Source: CAD feature listing. Evaluate the final solid. Frame: model axes, mm. A direction names the side the tool comes from. Give positions to 0.01 mm unless a question says otherwise; leave off trailing zeros. Loops run counter-clockwise (first coordinate to the right, second up) from the corner with the lowest first, then second, coordinate; pieces in that order, holes last. Notation, with made-up numbers: M -2.5,63.5 L 18.5,63.5 A15 ccw 18.5,74.5 Z; hole C -5.75,-31 d11. An arc over 180 degrees is marked long. Answer in a Markdown table with one row per item.
```python
from build123d import *

# Parameters (mm, degrees)
BOSS_EXTRUDE1_DEPTH                     = 580
TAP_DRILL_FOR_M10X1_25_TAP1_D           = 8.8
TAP_DRILL_FOR_M10X1_25_TAP1_CSINK_D     = 8.85
TAP_DRILL_FOR_M10X1_25_TAP1_CSINK_ANGLE = 90


with BuildPart() as part:
    # Sketch1 → Boss-Extrude1 (new body)
    with BuildSketch(Plane(origin=(0, 0, 0), x_dir=(1, 0, 0), z_dir=(0, 1, 0))):
        with BuildLine():
            Line((-28, 27.5), (0, 27.5))
            Line((0, 27.5), (0, -27.5))
            ThreePointArc((0, -27.5), (-1.464466094, -31.035533906), (-5, -32.5))
            Line((-5, -32.5), (-18, -32.5))
            Line((-18, -32.5), (-28, -22.5))
            Line((-28, -22.5), (-28, -3.5))
            Line((-28, -3.5), (-20, -3.5))
            Line((-20, -3.5), (-20, 12.5))
            Line((-20, 12.5), (-28, 12.5))
            Line((-28, 12.5), (-28, 27.5))
        make_face()
    extrude(amount=BOSS_EXTRUDE1_DEPTH)

    # Tap Drill for M10x1.25 Tap1 (through all)
    with Locations(Plane(origin=(0, 25, -4.5), x_dir=(0, 0, 1), z_dir=(1, 0, 0))):
        with Locations((0, 0), (0, -132.5), (0, -265), (0, -397.5), (0, -530)):
            CounterSinkHole(TAP_DRILL_FOR_M10X1_25_TAP1_D / 2, TAP_DRILL_FOR_M10X1_25_TAP1_CSINK_D / 2, counter_sink_angle=TAP_DRILL_FOR_M10X1_25_TAP1_CSINK_ANGLE)


solid = part.part
```
Q1. Mould query, pull axis Y, two halves, no side actions, for faces 3 (the cylindrical face through (-10.152, 285.637, -3.927)), 4 (the flat face through (-14, 0, 2)), 5 (the flat face through (-22.9, 285.9, 27.6)), 6 (the cylindrical face through (-10.152, 22.026, -1.257)). Classes: +Y half, -Y half, draft (parallel to the pull), parting line (faces both ways), or undercut.
Values follow:
| item | result |
|---|---|
| face 3 | undercut |
| face 4 | -Y half |
| face 5 | draft |
| face 6 | undercut |
Q2. Ray query, probe 1 along Y at (x, z) = (-5.25, -4.5); probe 2 along Z at (x, y) = (-12.5, 25); probe 3 along Z at (x, y) = (-4.75, 166.5). Return the intervals inside material, ascending. Write a range as from..to.
Values follow:
| item | result |
|---|---|
| probe 1 | 0..20.6, 29.4..153.1, 161.9..285.6, 294.4..418.1, 426.9..550.6, 559.4..580 |
| probe 2 | -27.5..-8.9, -0.1..32.5 |
| probe 3 | -27.5..32.49 |
Q3. Contact query for a flat-ended pin moving along its axis: pin 1 Ø11.5 at (y, z) = (157.5, -4.5) entering from -X. Output: stop coordinate, or through.
Values follow:
| item | result |
|---|---|
| pin 1 | x = -20 |
Q4. Reachability of faces 1 (the flat face through (-20, 286, -1)), 2 (the flat face through (-11, 286, 32.5)) from +Z, -Z, +X, -X, +Y, -Y: full face, straight path, thin tool, end or side. Return the list, or none.
Values follow:
| item | result |
|---|---|
| face 1 | -X, +Y, -Y |
| face 2 | +Z, +X, -X, +Y, -Y |
Q5. Section query A-A (y = 148). Output: boundary loops of the cut face in (x, z).
Values follow:
| item | result |
|---|---|
| outline | M -28,-27.5 L 0,-27.5 L 0,27.5 A5 ccw -5,32.5 L -18,32.5 L -28,22.5 L -28,3.5 L -20,3.5 L -20,-12.5 L -28,-12.5 Z |
